```python
from build123d import *

# Parameters (mm, degrees)
F1_DEPTH = 12.53708
F2_DEPTH = 148.17746
F3_DEPTH = 381


# Not quite as in the source:
# - ends of sketch curves that miss each other by under 0.0002 mm in the source are joined
# - a feature names something its author has since deleted; it is built from what else it names


with BuildPart() as f1:
    # F0 (on Front) → F1 (new body)
    with BuildSketch(Plane.XZ):
        with BuildLine():
            Line((-0.0432951165, 18.7523439527), (-62.6219127655, 18.7523439527))
            ThreePointArc((-62.6219127655, 18.7523439527), (-71.6021688866, 15.0326000737), (-75.3219127655, 6.0523439527))
            Line((-75.3219127655, 6.0523439527), (-75.3219127655, 0))
            Line((-75.3219127655, 0), (-65.1619127655, 0))
            add(Edge.make_bspline(
                [(-65.1619127655, 0), (-48.671609143, 3.823998258), (-23.9979293543, 18.7523570586), (-0.0432951165, 18.7523439527)],
                knots=[0, 0, 0, 0, 0.499698946, 0.499698946, 0.499698946, 0.499698946], degree=3))
        make_face()
        with BuildLine():
            add(Edge.make_bspline(
                [(-0.0432951165, 18.7523602083), (-0.0288631494, 18.7523602102), (23.9542012968, 18.7433586286), (47.2111099504, 3.7542823594), (65.1619127655, 0)],
                knots=[0.499698946, 0.499698946, 0.499698946, 0.499698946, 0.5, 1, 1, 1, 1], degree=3))
            add(Edge.make_bspline(
                [(-65.1619127655, 0), (-48.671609143, 3.823998258), (-23.9979293543, 18.7523570586), (-0.0432951165, 18.7523602083)],
                knots=[0, 0, 0, 0, 0.499698946, 0.499698946, 0.499698946, 0.499698946], degree=3))
            Line((-65.1619127655, 0), (-15.5171778125, 0))
            ThreePointArc((-15.5171778125, 0), (0, 15.5171778125), (15.5171778125, 0))
            Line((15.5171778125, 0), (65.1619127655, 0))
        make_face()
        with BuildLine():
            Line((62.6219127655, 18.7523439527), (-0.0432951165, 18.7523439527))
            add(Edge.make_bspline(
                [(-0.0432951165, 18.7523439527), (-0.0288631494, 18.7523602102), (23.9542012968, 18.7433586286), (47.2111099504, 3.7542823594), (65.1619127655, 0)],
                knots=[0.499698946, 0.499698946, 0.499698946, 0.499698946, 0.5, 1, 1, 1, 1], degree=3))
            Line((65.1619127655, 0), (75.3219127655, 0))
            Line((75.3219127655, 0), (75.3219127655, 6.0523439527))
            ThreePointArc((75.3219127655, 6.0523439527), (71.6021688866, 15.0326000737), (62.6219127655, 18.7523439527))
        make_face()
        with BuildLine():
            add(Edge.make_bspline(
                [(-65.1619127655, 0), (-48.671609143, -3.823998258), (-23.9979293543, -18.7523570586), (-0.0432951165, -18.7523602083)],
                knots=[0, 0, 0, 0, 0.499698946, 0.499698946, 0.499698946, 0.499698946], degree=3))
            Line((-65.1619127655, 0), (-75.3219127655, 0))
            Line((-75.3219127655, 0), (-75.3219127655, -6.0523439527))
            ThreePointArc((-75.3219127655, -6.0523439527), (-71.6021688866, -15.0326000737), (-62.6219127655, -18.7523439527))
            Line((-62.6219127655, -18.7523439527), (-0.0432951165, -18.7523602083))
        make_face()
        with BuildLine():
            Line((-15.5171778125, 0), (-65.1619127655, 0))
            add(Edge.make_bspline(
                [(-65.1619127655, 0), (-48.671609143, -3.823998258), (-23.9979293543, -18.7523570586), (-0.0432951165, -18.7523602083)],
                knots=[0, 0, 0, 0, 0.499698946, 0.499698946, 0.499698946, 0.499698946], degree=3))
            add(Edge.make_bspline(
                [(-0.0432951165, -18.7523602083), (-0.0288631494, -18.7523602102), (23.9542012968, -18.7433586286), (47.2111099504, -3.7542823594), (65.1619127655, 0)],
                knots=[0.499698946, 0.499698946, 0.499698946, 0.499698946, 0.5, 1, 1, 1, 1], degree=3))
            Line((65.1619127655, 0), (15.5171778125, 0))
            ThreePointArc((15.5171778125, 0), (0, -15.5171778125), (-15.5171778125, 0))
        make_face()
        with BuildLine():
            Line((75.3219127655, 0), (65.1619127655, 0))
            add(Edge.make_bspline(
                [(-0.0432951165, -18.7523602083), (-0.0288631494, -18.7523602102), (23.9542012968, -18.7433586286), (47.2111099504, -3.7542823594), (65.1619127655, 0)],
                knots=[0.499698946, 0.499698946, 0.499698946, 0.499698946, 0.5, 1, 1, 1, 1], degree=3))
            Line((-0.0432951165, -18.7523602083), (62.6219127655, -18.7523439527))
            ThreePointArc((62.6219127655, -18.7523439527), (71.6021688866, -15.0326000737), (75.3219127655, -6.0523439527))
            Line((75.3219127655, -6.0523439527), (75.3219127655, 0))
        make_face()
        with BuildLine():
            ThreePointArc((15.5171778125, 0), (0, 15.5171778125), (-15.5171778125, 0))
            ThreePointArc((-15.5171778125, 0), (0, -15.5171778125), (15.5171778125, 0))
        make_face()
    extrude(amount=-F1_DEPTH)

    # F0 (on Front) → F2 (join)
    with BuildSketch(Plane.XZ):
        with BuildLine():
            ThreePointArc((15.5171778125, 0), (0, 15.5171778125), (-15.5171778125, 0))
            ThreePointArc((-15.5171778125, 0), (0, -15.5171778125), (15.5171778125, 0))
        make_face()
    extrude(amount=-F2_DEPTH)

    # F0 (on Front) → F3 (join)
    with BuildSketch(Plane.XZ):
        with BuildLine():
            add(Edge.make_bspline(
                [(-0.0432951165, 18.7523602083), (-0.0288631494, 18.7523602102), (23.9542012968, 18.7433586286), (47.2111099504, 3.7542823594), (65.1619127655, 0)],
                knots=[0.499698946, 0.499698946, 0.499698946, 0.499698946, 0.5, 1, 1, 1, 1], degree=3))
            add(Edge.make_bspline(
                [(-65.1619127655, 0), (-48.671609143, 3.823998258), (-23.9979293543, 18.7523570586), (-0.0432951165, 18.7523602083)],
                knots=[0, 0, 0, 0, 0.499698946, 0.499698946, 0.499698946, 0.499698946], degree=3))
            Line((-65.1619127655, 0), (-15.5171778125, 0))
            ThreePointArc((-15.5171778125, 0), (0, 15.5171778125), (15.5171778125, 0))
            Line((15.5171778125, 0), (65.1619127655, 0))
        make_face()
        with BuildLine():
            Line((-15.5171778125, 0), (-65.1619127655, 0))
            add(Edge.make_bspline(
                [(-65.1619127655, 0), (-48.671609143, -3.823998258), (-23.9979293543, -18.7523570586), (-0.0432951165, -18.7523602083)],
                knots=[0, 0, 0, 0, 0.499698946, 0.499698946, 0.499698946, 0.499698946], degree=3))
            add(Edge.make_bspline(
                [(-0.0432951165, -18.7523602083), (-0.0288631494, -18.7523602102), (23.9542012968, -18.7433586286), (47.2111099504, -3.7542823594), (65.1619127655, 0)],
                knots=[0.499698946, 0.499698946, 0.499698946, 0.499698946, 0.5, 1, 1, 1, 1], degree=3))
            Line((65.1619127655, 0), (15.5171778125, 0))
            ThreePointArc((15.5171778125, 0), (0, -15.5171778125), (-15.5171778125, 0))
        make_face()
        with BuildLine():
            ThreePointArc((15.5171778125, 0), (0, 15.5171778125), (-15.5171778125, 0))
            ThreePointArc((-15.5171778125, 0), (0, -15.5171778125), (15.5171778125, 0))
        make_face()
    extrude(amount=F3_DEPTH)


solid = f1.part
```
Model file for the job. Use its own axes, mm. A direction names the side the tool comes from. Give positions to 0.01 mm unless a question says otherwise; leave off trailing zeros. Loops run counter-clockwise (first coordinate to the right, second up) from the corner with the lowest first, then second, coordinate; pieces in that order, holes last. Notation, with made-up numbers: (25, -17) -> (56, -17) arc R20 cw to (56, 2) -> close; hole circle Ø5 at (20, 78.25). An arc over 180 degrees is marked (long way). Use CSV: the item, a comma, the result in double quotes. Start each with the question number.
1) Flat gauge pins, fed straight in: pin 1 Ø6 at (y, z) = (87.5, -5) entering from -X; pin 2 Ø12 at (y, z) = (55.5, 9) entering from +X; pin 3 Ø4 at (x, z) = (-54, 8) entering from -Y. Where does each tip first touch, or does it go through?
2) Wall check: line 1 (Y direction, x = 68, z = -14.5); line 2 (Y direction, x = -9, z = 17); line 3 (Z direction, x = 1, y = -105). Give the ranges that are in metal, low to high.
3) Slice it at A-A on y = 40. Give the cut face in (x, z).
4) Tool access for faces 1 (the cylindrical face through (2.02, 79.408, -15.385)), 2 (the flat face through (32, 6, 18.752)), 3 (the flat face through (54, 0, 4)), 4 (the flat face through (-55, 0, 4)): list every direction of +Z, -Z, +X, -X, +Y, -Y with a clear straight run to the whole face (end or side of a thin tool).
Computed values:
1,pin 1,"stops at x = -15.39"
1,pin 2,"stops at x = 15.22"
1,pin 3,"stops at y = 0"
2,line 1,"y = 0 to 12.54"
2,line 2,"y = -381 to 12.54"
2,line 3,"z = -18.74 to 18.74"
3,outline,"circle Ø31.03 at (0, 0)"
4,face 1,"+Y"
4,face 2,"+Z, +X, -X, +Y, -Y"
4,face 3,"+X, -Y"
4,face 4,"-X, -Y"
